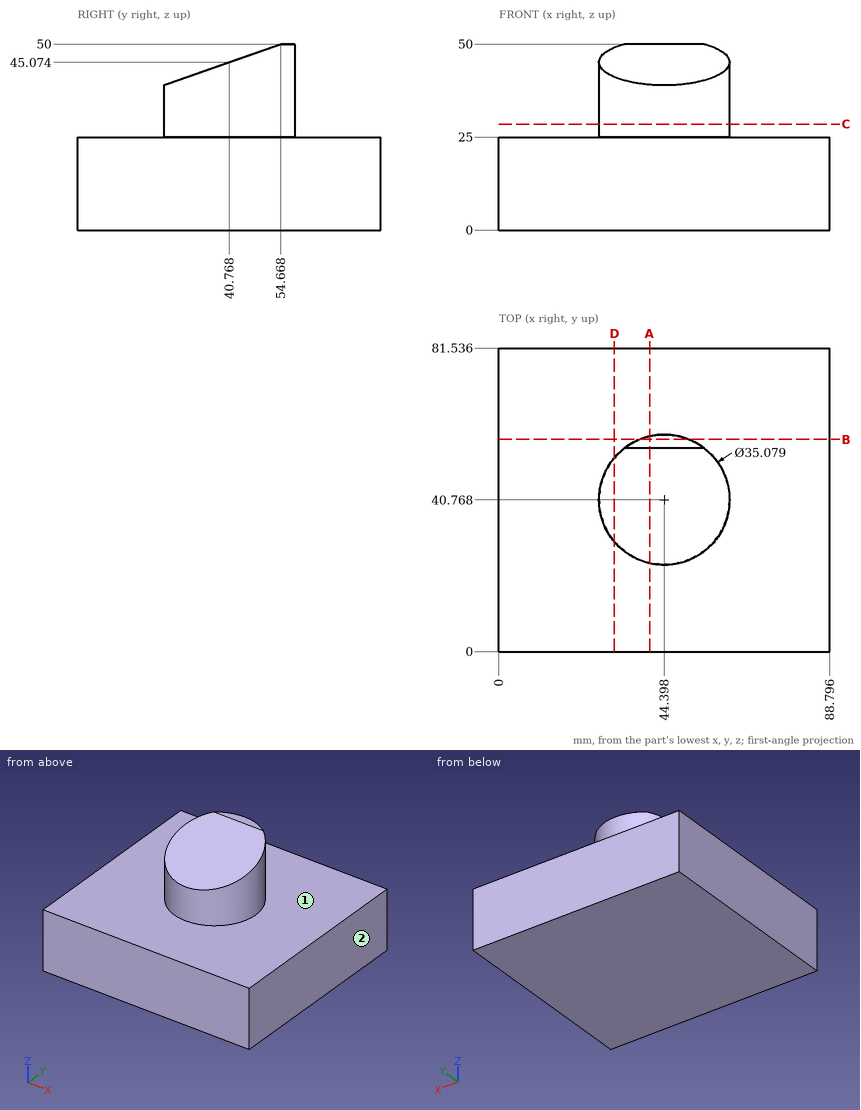
Here's the drawing with two shaded views (mm, measured from the low corner). I have some questions. A direction names the side the tool comes from. Give positions to 0.01 mm unless a question says otherwise; leave off trailing zeros. Order: outer loops, then holes, each group sorted by start corner. A loop starts at its lowest first (then second) coordinate and runs counter-clockwise, first axis right, second up. Notation, with made-up numbers: (29.25, 78.5) -> (63.25, 78.5) arc R14 ccw to (63.25, 105.5) -> close; hole circle Ø9 at (-8, 68.5). An arc over 180 degrees is marked (long way). Use a Markdown table: item, result. Add a question column.
Item 1: Imagine slicing it at C-C on z = 28.5. Please give me the cut outline in (x, y).
Item 2: Imagine slicing it at A-A on x = 40.5. Please give me the cut outline in (y, z) (1 decimal).
Item 3: Will these pins go through, and if not, where does the flat tip stop? pin 1 (6 mm diameter, centred on x = 35, y = 21.5, fed in from +Z); pin 2 (8 mm diameter, centred on y = 33.5, z = 42, fed in from -X).
Item 4: Imagine slicing it at B-B on y = 57. Please give me the cut outline in (x, z) (1 decimal).
Item 5: I need wall thicknesses on line 1 (Z direction, x = 11, y = 10.5); line 2 (Z direction, x = 54, y = 35); line 3 (X direction, y = 25, z = 29) (1 decimal). Which ranges of each line are inside material? Lowest first, please.
Item 6: Imagine slicing it at D-D on x = 31. Please give me the cut outline in (y, z) (1 decimal), plus the area to 3 significant figures.
Item 7: For the marked faces 1 and 2, which set-ups out of +Z, -Z, +X, -X, +Y, -Y let a thin tool reach every point of the face, with its end or its side?
Data:
| question | item | result |
|---|---|---|
| 1 | outline | circle Ø35.08 at (44.4, 40.77) |
| 2 | outline | (0, 0) -> (81.5, 0) -> (81.5, 25) -> (57.9, 25) -> (57.9, 50) -> (54.7, 50) -> (23.7, 39) -> (23.7, 25) -> (0, 25) -> close |
| 3 | pin 1 | stops at z = 25 |
| 3 | pin 2 | stops at x = 27.17 |
| 4 | outline | (0, 0) -> (88.8, 0) -> (88.8, 25) -> (51, 25) -> (51, 50) -> (37.8, 50) -> (37.8, 25) -> (0, 25) -> close |
| 5 | line 1 | z = 0 to 25 |
| 5 | line 2 | z = 0 to 43.03 |
| 5 | line 3 | x = 36.7 to 52.1 |
| 6 | outline | (0, 0) -> (81.5, 0) -> (81.5, 25) -> (52.1, 25) -> (52.1, 49.1) -> (29.4, 41.1) -> (29.4, 25) -> (0, 25) -> close |
| 6 | area | 2,490 mm² |
| 7 | face 1 | +Z |
| 7 | face 2 | +Z, -Z, +X, +Y, -Y |
